Could you check a few things on this model? Use its own coordinates, in mm. A direction names the side the tool comes from. Coordinates: 2 decimals unless noted, no trailing zeros. Loops run counter-clockwise (first coordinate to the right, second up) from the corner with the lowest first, then second, coordinate; pieces in that order, holes last. Notation, with made-up numbers: (-18, -37.75) - (14, -37.75) arc R16 cw to (14, -25.75) - close; hole circle Ø1 at (-1, 23.25). An arc over 180 degrees is marked (long way). Put each result on its own line as item: value. Start each with the question number.
Autodesk Inventor part; units mm, degrees
ref_plane "YZ Plane" through (0, 0, 0) normal (1, 0, 0) x (0, 1, 0)
ref_plane "XZ Plane" through (0, 0, 0) normal (0, 1, 0) x (-1, 0, 0)
ref_plane "XY Plane" through (0, 0, 0) normal (0, 0, 1) x (1, 0, 0)
sketch "Эскиз1" plane through (0, 0, 0) normal (0, 0, 1) x (1, 0, 0)
  circle A0 centre (0, 0) radius 5
  circle A1 centre (0, 0) radius 20.7
  line L0 (0, -28.98) -> (0, 28.98) construction
  line L1 (-28.98, 0) -> (28.98, 0) construction
  line L2 (2.3094, 8) -> (-2.3094, 8)
  line L3 (-2.3094, 8) -> (-4.6188, 12)
  line L4 (-4.6188, 12) -> (-2.3094, 16)
  line L5 (-2.3094, 16) -> (2.3094, 16)
  line L6 (2.3094, 16) -> (4.6188, 12)
  line L7 (4.6188, 12) -> (2.3094, 8)
  line L8 (-8.0829, -10) -> (-12.7017, -10)
  line L9 (-5.7735, -6) -> (-8.0829, -10)
  line L10 (-8.0829, -2) -> (-5.7735, -6)
  line L11 (-12.7017, -2) -> (-8.0829, -2)
  line L12 (-15.0111, -6) -> (-12.7017, -2)
  line L13 (-12.7017, -10) -> (-15.0111, -6)
  line L14 (12.7017, -2) -> (15.0111, -6)
  line L15 (8.0829, -2) -> (12.7017, -2)
  line L16 (5.7735, -6) -> (8.0829, -2)
  line L17 (8.0829, -10) -> (5.7735, -6)
  line L18 (12.7017, -10) -> (8.0829, -10)
  line L19 (15.0111, -6) -> (12.7017, -10)
  point P0 (0, 12)
  dimension "d0" = 10
  dimension "d1" = 41.4
  dimension "d10" = 12
  dimension "d11" = 8
  dimension "d14" = 360
extrude "Выдавливание1" add sketch "Эскиз1" along normal blind 4
properties part number "Бортик внутренний (конусной катушки)"
(1) If we mould it in two halves opening along X, with no side actions, what happens to faces 3 (the flat face through (6.944, -8.028, 1.972)), 4 (the flat face through (4, -4, 4))? For each: pulls with the +X half, pulls with the -X half, needs draft (parallel to the pull), parting line crosses it, or undercut.
(2) For pin 1 Ø2 at (x, z) = (-11, 1.5) entering from +Y; pin 2 Ø2 at (x, z) = (1, 3.5) entering from +Y; pin 3 Ø2 at (x, z) = (-11, 1) entering from -Y, each with a flat end and sliding along its axis, tell me the tip position at first contact or that it passes through.
(3) I need wall thicknesses on L1, parallel to Y at x = 0, z = 1.4; L2, parallel to X at y = -6.5, z = 0.55; L3, parallel to Y at x = 3, z = 0.2. Which ranges of each line are inside material? Lowest first, please. Write a range as [from, to].
(4) I want a section at A-A on x = 0. List the corners of the cut face in (y, z) for me.
(5) I want a section at C-C on z = 1. List the corners of the cut face in (x, y) for me, and give its area (3 significant figures).
(6) I want a section at D-D on x = -12. List the corners of the cut face in (y, z) for me.
(7) I want a section at B-B on y = 0. List the corners of the cut face in (x, z) for me, and give its area (3 significant figures).
(8) Which directions (+Z, -Z, +X, -X, +Y, -Y) give clear straight access to the entire face, cutting with the end or side of a thin tool? Please do faces 1 (the flat face through (4, -4, 0)), 2 (the flat face through (-6.944, -3.972, 1.972)).
Answer sheet:
1. face 3: undercut
1. face 4: needs draft
2. pin 1: stops at y = 18.12
2. pin 2: stops at y = 20.7
2. pin 3: stops at y = -18.12
3. L1: y = [-20.7, -5], [5, 8], [16, 20.7]
3. L2: x = [-19.65, -14.72], [-6.06, 6.06], [14.72, 19.65]
3. L3: y = [-20.48, -4], [4, 9.2], [14.8, 20.48]
4. outline: (-20.7, 0) - (-5, 0) - (-5, 4) - (-20.7, 4) - close; (5, 0) - (8, 0) - (8, 4) - (5, 4) - close; (16, 0) - (20.7, 0) - (20.7, 4) - (16, 4) - close
5. outline: circle Ø41.4 at (0, 0); hole (-15.01, -6) - (-12.7, -10) - (-8.08, -10) - (-5.77, -6) - (-8.08, -2) - (-12.7, -2) - close; hole circle Ø10 at (0, 0); hole (-4.62, 12) - (-2.31, 8) - (2.31, 8) - (4.62, 12) - (2.31, 16) - (-2.31, 16) - close; hole (5.77, -6) - (8.08, -10) - (12.7, -10) - (15.01, -6) - (12.7, -2) - (8.08, -2) - close
5. area: 1,100 mm^2
6. outline: (-16.87, 0) - (-10, 0) - (-10, 4) - (-16.87, 4) - close; (-2, 0) - (16.87, 0) - (16.87, 4) - (-2, 4) - close
7. outline: (-20.7, 0) - (-5, 0) - (-5, 4) - (-20.7, 4) - close; (5, 0) - (20.7, 0) - (20.7, 4) - (5, 4) - close
7. area: 126 mm^2
8. face 1: -Z, +X, -X, +Y, -Y
8. face 2: +Z, -Z
